Build history of the part. All positions in model axes, mm. Give positions to 0.01 mm unless a question says otherwise; leave off trailing zeros. Order: outer loops, then holes, each group sorted by start corner. A loop starts at its lowest first (then second) coordinate and runs counter-clockwise, first axis right, second up. Notation, with made-up numbers: (-21.5, 8) - (22.5, 8) arc R13 cw to (22.5, 25) - close; hole circle Ø5 at (-33, 12.25). An arc over 180 degrees is marked (long way). One line per item, written item: value.
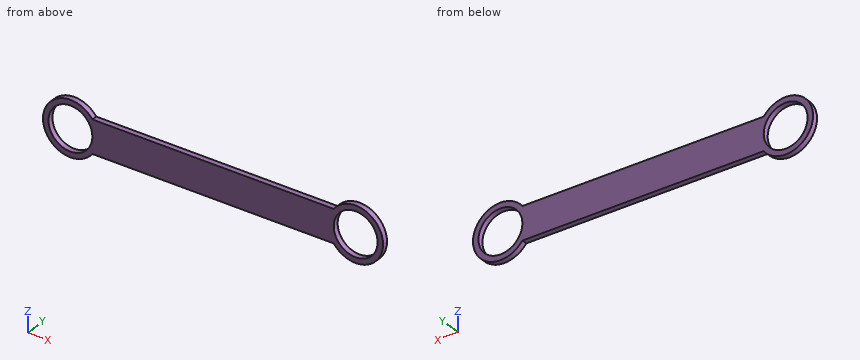
```python
from build123d import *

# Parameters (mm, degrees)
F0_R     = 25.4
F1_DEPTH = 6.35


with BuildPart() as f1:
    # F0 (on Front) → F1 (new body)
    with BuildSketch(Plane.XZ):
        with BuildLine():
            ThreePointArc((-42.59572, -10.614441), (-37.875025, -1.604672), (-36.24572, 8.435559))
            ThreePointArc((-36.24572, 8.435559), (-37.875025, 18.475791), (-42.59572, 27.485559))
            ThreePointArc((-42.59572, 27.485559), (-99.74572, 8.435559), (-42.59572, -10.614441))
        make_face()
        with Locations((-67.99572, 8.435559)):
            Circle(F0_R, mode=Mode.SUBTRACT)
        with BuildLine():
            ThreePointArc((-42.59572, 27.485559), (-37.875025, 18.475791), (-36.24572, 8.435559))
            ThreePointArc((-36.24572, 8.435559), (-37.875025, -1.604672), (-42.59572, -10.614441))
            Line((-42.59572, -10.614441), (236.80428, -10.614441))
            ThreePointArc((236.80428, -10.614441), (230.45428, 8.435559), (236.80428, 27.485559))
            Line((236.80428, 27.485559), (97.10428, 27.485559))
            Line((97.10428, 27.485559), (-42.59572, 27.485559))
        make_face()
        with BuildLine():
            ThreePointArc((236.80428, 27.485559), (230.45428, 8.435559), (236.80428, -10.614441))
            ThreePointArc((236.80428, -10.614441), (272.244512, -21.685135), (293.95428, 8.435559))
            ThreePointArc((293.95428, 8.435559), (272.244512, 38.556254), (236.80428, 27.485559))
        make_face()
        with Locations((262.20428, 8.435559)):
            Circle(F0_R, mode=Mode.SUBTRACT)
    extrude(amount=F1_DEPTH)


solid = f1.part
```
(1) Slice it at C-C, the plane x = 76. Give the cut face in (y, z).
Completed:
outline: (-6.35, -10.61) - (0, -10.61) - (0, 27.49) - (-6.35, 27.49) - close
(2) Slice it at B-B, the plane y = -4.75. Give the cut face in (x, z), and give its area (3 significant figures).
Completed:
outline: (-42.6, -10.61) - (236.8, -10.61) arc R31.75 ccw (long way) to (236.8, 27.49) - (-42.6, 27.49) arc R31.75 ccw (long way) to start; hole circle Ø50.8 at (-68, 8.44); hole circle Ø50.8 at (262.2, 8.44)
area: 12,600 mm²
(3) Pin check, flat tips, straight feed: P1, Ø3, axis at y = -4.5, z = -4, coming from the -X side; P2, Ø1.5, axis at x = 31, y = -5.5, coming from the +Z side. Stop position of each tip, or through.
Completed:
P1: x = -97.8
P2: z = 27.49
(4) Slice it at D-D, the plane z = 14.5. Give the cut face in (x, y), and give its area (3 significant figures).
Completed:
outline: (-99.16, -6.35) - (-92.66, -6.35) - (-92.66, 0) - (-99.16, 0) - close; (-43.33, -6.35) - (237.54, -6.35) - (237.54, 0) - (-43.33, 0) - close; (286.87, -6.35) - (293.37, -6.35) - (293.37, 0) - (286.87, 0) - close
area: 1,870 mm²
(5) Drill centre lines: line 1 (X direction, y = -0.5, z = -7.5); line 2 (X direction, y = -2.75, z = -11.5); line 3 (X direction, y = -5.5, z = -8.5). Where is each one in solid material? Low to high.
Completed:
line 1: -95.46 to -87.77, -48.22 to 242.43, 281.98 to 289.67
line 2: -92.71 to -83.74, -52.26 to -43.28, 237.49 to 246.46, 277.94 to 286.92
line 3: -94.85 to -86.93, -49.07 to 243.27, 281.13 to 289.06
(6) Slice it at A-A, the plane z = 0.5. Give the cut face in (x, y), and give its area (3 significant figures).
Completed:
outline: (-98.74, -6.35) - (-92.12, -6.35) - (-92.12, 0) - (-98.74, 0) - close; (-43.87, -6.35) - (238.08, -6.35) - (238.08, 0) - (-43.87, 0) - close; (286.33, -6.35) - (292.95, -6.35) - (292.95, 0) - (286.33, 0) - close
area: 1,870 mm²
